Build history of the part. All positions in model axes, mm. A direction names the side the tool comes from. Give positions to 0.01 mm unless a question says otherwise; leave off trailing zeros. Loops run counter-clockwise (first coordinate to the right, second up) from the corner with the lowest first, then second, coordinate; pieces in that order, holes last. Notation, with made-up numbers: M 21,-4 L 42,-4 A30 ccw 42,23 Z; hole C -15,2.25 d10. An arc over 180 degrees is marked long. Answer as a JSON object with one key per item and string values. Group by question number.
1. Slice it at A-A (x = 0). List the corners of the cut face in (y, z), then the cut area to 3 significant figures.
2. Drop flat-ended pins along their axis: pin 1 Ø3 at (y, z) = (44.5, 76.5) entering from -X; pin 2 Ø6 at (y, z) = (38.5, 218) entering from -X; pin 3 Ø8 at (x, z) = (30, 61.5) entering from +Y. Give the stop position or say it passes through.
3. Slice it at C-C (y = 27). List the corners of the cut face in (x, z), then the cut area to 3 significant figures.
4. Slice it at B-B (z = 162). List the corners of the cut face in (x, y).
5. 3-axis set-ups, long thin cutter, end or side, ignore diameter. For faces 1 (the face through (26, -54, 304.8)), 2 (the face through (-1, -89, 101.6)): which of +Z, -Z, +X, -X, +Y, -Y reach the whole face in a straight line?
6. Slice it at D-D (z = 83). List the corners of the cut face in (x, y), then the cut area to 3 significant figures.
7. Drill centre lines: line 1 along X through (y, z) = (0, 242); line 2 along Z through (x, y) = (17.5, -110); line 3 along Y through (x, z) = (16.5, 215). Where is each one in solid material? Low to high. Write a range as [from, to].
from build123d import *

# Parameters (mm, degrees)
F1_DEPTH = 304.8
F2_DEPTH = 101.6


with BuildPart() as f1:
    # F0 (on Top) → F1 (new body)
    with BuildSketch(Plane.XY):
        with BuildLine():
            ThreePointArc((55.88, -111.210239), (105.936576, -65.327891), (124.46, 0))
            ThreePointArc((124.46, 0), (-65.327891, 105.936576), (-55.88, -111.210239))
            Line((-55.88, -111.210239), (-55.88, 0))
            ThreePointArc((-55.88, 0), (0, 55.88), (55.88, 0))
            Line((55.88, 0), (55.88, -111.210239))
        make_face()
        with BuildLine():
            Line((-55.88, 0), (-55.88, -111.210239))
            ThreePointArc((-55.88, -111.210239), (0, -124.46), (55.88, -111.210239))
            Line((55.88, -111.210239), (55.88, 0))
            ThreePointArc((55.88, 0), (0, -55.88), (-55.88, 0))
        make_face()
    extrude(amount=F1_DEPTH)

    # F0 (on Top) → F2 (cut)
    with BuildSketch(Plane.XY):
        with BuildLine():
            Line((-55.88, 0), (-55.88, -111.210239))
            ThreePointArc((-55.88, -111.210239), (0, -124.46), (55.88, -111.210239))
            Line((55.88, -111.210239), (55.88, 0))
            ThreePointArc((55.88, 0), (0, -55.88), (-55.88, 0))
        make_face()
    extrude(amount=F2_DEPTH, mode=Mode.SUBTRACT)


solid = f1.part
Established:
{
 "1": {"outline": "M -124.46,101.6 L -55.88,101.6 L -55.88,304.8 L -124.46,304.8 Z; M 55.88,0 L 124.46,0 L 124.46,304.8 L 55.88,304.8 Z", "area": "34,800 mm^2"},
 "2": {"pin 1": "stops at x = -116.8", "pin 2": "stops at x = -119.29", "pin 3": "stops at y = 121.71"},
 "3": {"outline": "M -121.5,0 L -48.92,0 L -48.92,304.8 L -121.5,304.8 Z; M 48.92,0 L 121.5,0 L 121.5,304.8 L 48.92,304.8 Z", "area": "44,200 mm^2"},
 "4": {"outline": "M -55.88,-111.21 A124.46 ccw 55.88,-111.21 A124.46 ccw 124.46,0 A124.46 ccw long Z; hole C 0,0 d111.76"},
 "5": {"face 1": "+Z, +X, -X, +Y, -Y", "face 2": "-Z, -Y"},
 "6": {"outline": "M -55.88,-111.21 L -55.88,0 A55.88 cw 55.88,0 L 55.88,-111.21 A124.46 ccw 124.46,0 A124.46 ccw long Z", "area": "30,300 mm^2"},
 "7": {"line 1": "x = [-124.46, -55.88], [55.88, 124.46]", "line 2": "z = [101.6, 304.8]", "line 3": "y = [-123.36, -53.39], [53.39, 123.36]"}
}
